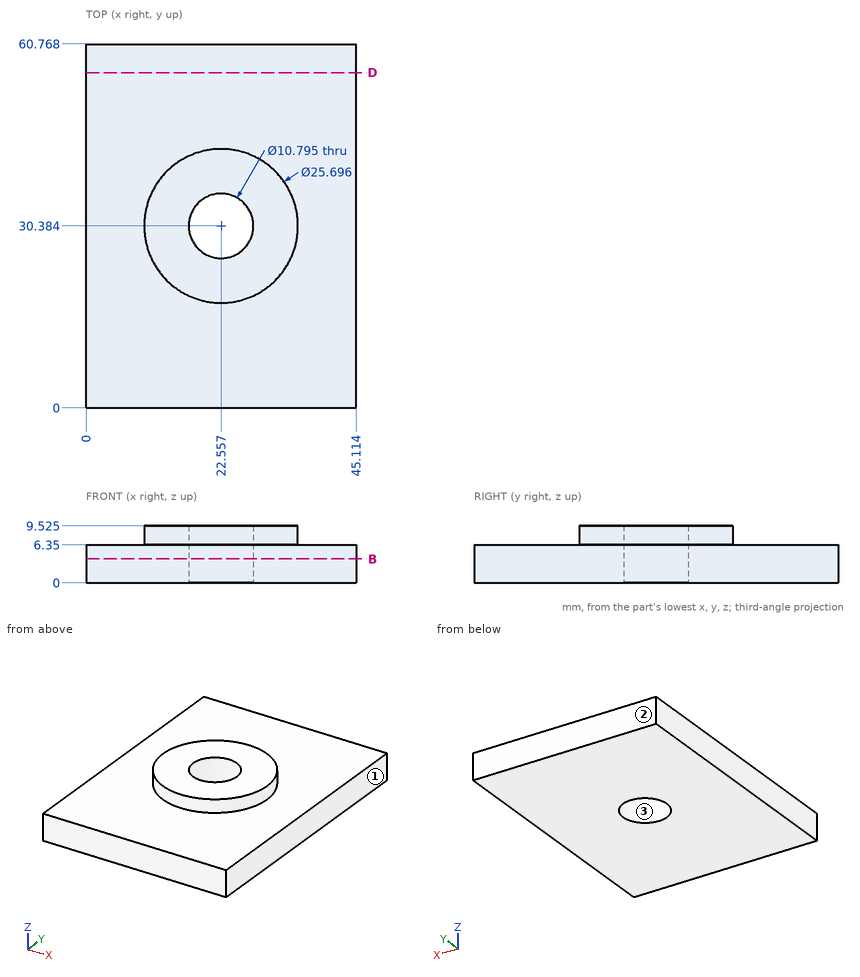
Answer from the drawing. Dimensions are ordinates in mm from the lowest x, y and z of the part. Coordinates: 2 decimals unless noted, no trailing zeros. Loops run counter-clockwise (first coordinate to the right, second up) from the corner with the lowest first, then second, coordinate; pieces in that order, holes last.
1) Section D-D (y = 56) is taken. Give the vertices of the cut face in (x, z).
Results:
outline: (0, 0) - (45.11, 0) - (45.11, 6.35) - (0, 6.35) - close
2) For a pull along X with two mould halves and no side action, classify the marked faces 1, 2 and 3 as +X half, -X half, draft (parallel to the pull), parting line (faces both ways), or undercut.
Results:
face 1: +X half
face 2: draft
face 3: undercut
3) Consider probe 1 along Z at (x, y) = (2, 33.5); probe 2 along Y at (x, z) = (26.5, 1.75); probe 3 along Y at (x, z) = (23.5, 7.25). Determine where each line is inside the solid, lowest interval first.
Results:
probe 1: z = 0 to 6.35
probe 2: y = 0 to 26.7, 34.07 to 60.77
probe 3: y = 17.57 to 25.07, 35.7 to 43.2
4) Section B-B (z = 4) is taken. Give the vertices of the cut face in (x, y) (1 decimal).
Results:
outline: (0, 0) - (45.1, 0) - (45.1, 60.8) - (0, 60.8) - close; hole circle Ø10.8 at (22.6, 30.4)
